from build123d import *

# Parameters (mm, degrees)
F0_R     = 12.065
F1_DEPTH = 10.795
F2_R     = 7.9375
F3_DEPTH = 1.905
F4_R     = 3.175
F5_DEPTH = 3.302
F7_D     = 2.7051
F9_D     = 2.3749
F9_DEPTH = 12.066


with BuildPart() as f1:
    # F0 (on Front) → F1 (new body)
    with BuildSketch(Plane.XZ):
        Circle(F0_R)
    extrude(amount=F1_DEPTH)

    # F2 (on face) → F3 (cut)
    with BuildSketch(Plane.XZ):
        Circle(F2_R)
    extrude(amount=F3_DEPTH, mode=Mode.SUBTRACT)

    # F4 (on face) → F5 (cut)
    with BuildSketch(Plane.XZ):
        Circle(F4_R)
    extrude(amount=F5_DEPTH, mode=Mode.SUBTRACT)

    # F7 (through all)
    with Locations(Plane.XZ.offset(10.795)):
        with Locations((0, 0)):
            Hole(F7_D / 2)

    # F9 (through all, one way)
    with BuildSketch(Plane(origin=(0, 0, 0), x_dir=(0, 1, 0), z_dir=(-1, 0, 0))):
        with Locations((-4.7127064317, 0)):
            Circle(F9_D / 2)
    extrude(amount=-F9_DEPTH, mode=Mode.SUBTRACT)


solid = f1.part
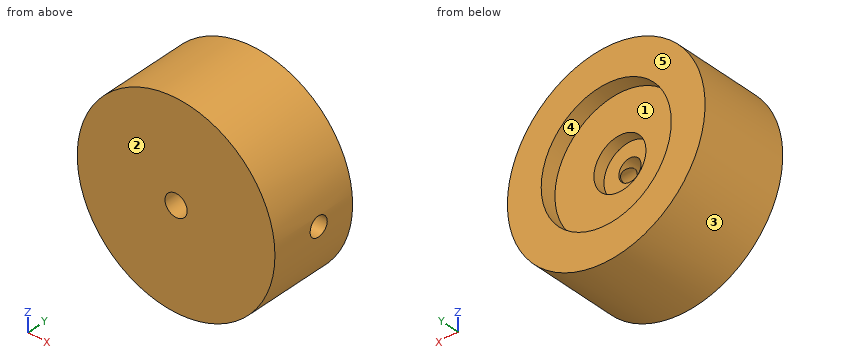
Could you check a few things on this model? Use its own coordinates, in mm. Face numbers are marked on the shaded views. A direction names the side the tool comes from. Give positions to 0.01 mm unless a question says otherwise; leave off trailing zeros. Order: outer loops, then holes, each group sorted by start corner. A loop starts at its lowest first (then second) coordinate and runs counter-clockwise, first axis right, second up.
1. Suppose I cut it at D-D (y = -9.75). Write out the boundary of the cut face in (x, z) (3 decimals).
Answers below:
outline: circle Ø24.13 at (0, 0); hole circle Ø2.705 at (0, 0)
2. Thinking about a two-plate mould opening in X: for the marked faces 3, 4 and 5, which applies, +X half, -X half, draft (parallel to the pull), parting line (faces both ways), or undercut?
Answers below:
face 3: parting line
face 4: undercut
face 5: draft
3. Suppose I cut it at B-B (x = 0). Write out the boundary of the cut face in (y, z) (1 decimal).
Answers below:
outline: (-10.8, -12.1) - (0, -12.1) - (0, -7.9) - (-1.9, -7.9) - (-1.9, -3.2) - (-3.3, -3.2) - (-3.3, -1.4) - (-10.8, -1.4) - close; (-10.8, 1.4) - (-3.3, 1.4) - (-3.3, 3.2) - (-1.9, 3.2) - (-1.9, 7.9) - (0, 7.9) - (0, 12.1) - (-10.8, 12.1) - close
4. I need wall thicknesses on L1, parallel to Z at x = 0, y = -2.8 (3 decimals); L2, parallel to Z at x = 0, y = -0.85 (1 decimal); L3, parallel to Y at x = -3.5, z = 5 (3 decimals). Which ranges of each line are inside material? Lowest first, please.
Answers below:
L1: z = -12.065 to -3.175, 3.175 to 12.065
L2: z = -12.1 to -7.9, 7.9 to 12.1
L3: y = -10.795 to -1.905
5. For pin 1 (3 mm diameter, centred on x = -2, y = -5.5, fed in from -Z); pin 2 (1 mm diameter, centred on y = -9.5, z = -7, fed in from -X); pin 3 (8.5 mm diameter, centred on x = 0, z = 0, fed in from +Y) (3 decimals), each with a flat end and sliding along its axis, tell me the tip position at first contact or that it passes through.
Answers below:
pin 1: stops at z = -12.05
pin 2: stops at x = -10.16
pin 3: stops at y = -1.905
6. Which directions (+Z, -Z, +X, -X, +Y, -Y) give clear straight access to the entire face, cutting with the end or side of a thin tool? Please do the marked faces 1 and 2.
Answers below:
face 1: +Y
face 2: +Z, -Z, +X, -X, -Y
7. Suppose I cut it at A-A (z = 0). State how many separate pieces and enclosed holes the cut face has, plus the area to 3 significant figures.
Answers below:
separate pieces: 3
enclosed holes: 0
area: 176 mm2
8. Suppose I cut it at C-C (x = 5.5). Write out the boundary of the cut face in (y, z) (3 decimals), plus the area to 3 significant figures.
Answers below:
outline: (-10.795, -10.738) - (0, -10.738) - (0, -5.723) - (-1.905, -5.723) - (-1.905, 5.723) - (0, 5.723) - (0, 10.738) - (-10.795, 10.738) - close; hole circle Ø2.375 at (-4.713, 0)
area: 206 mm2
